Build history of the part. All positions in model axes, mm. A direction names the side the tool comes from. Round coordinates to 2 decimals unless told otherwise and drop trailing zeros. Write each loop counter-clockwise with the first axis right and the second up, starting at its lowest first coordinate (ties: lowest second). Pieces come first, ordered by that corner, then holes. Notation, with made-up numbers: M 53.5,65 L 84.5,65 A12 ccw 84.5,82 Z; hole C -31,39 d8. An arc over 180 degrees is marked long. Write item = value, one per line.
Autodesk Fusion 360 part; units mm, degrees
sketch "Sketch1" plane through (0, 0, 0) normal (0, 1, 0) x (1, 0, 0)
  circle A0 centre (0, 0) radius 12.5
  dimension "d1" = 25
extrude "Extrude1" add sketch "Sketch1" along normal blind 3 makes body 1
chamfer "Chamfer1" distance 3 angle 45 1 edges at (-11.6541, 3, 4.5202) on bodies 1
sketch "Sketch2" plane through (0, 3, 0) normal (0, 1, 0) x (-1, 0, 0)
  circle A0 centre (0, 0) radius 9.5
  circle A1 centre (0, 0) radius 12.5
  dimension "d5" = 25
extrude "Extrude2" add sketch "Sketch2" along normal blind 1 contours A0 | A1 bodies 1
sketch "Sketch3" plane through (0, 0, 0) normal (0, 0, 1) x (1, 0, 0)
  line L0 (0, 0) -> (0.5, 0)
  line L1 (0.5, 0) -> (0.5, 3)
  line L2 (0.5, 3) -> (0, 3)
  line L3 (0, 3) -> (0, 0)
  line L4 (12.5, 3) -> (-12.5, 3)
extrude "Extrude3" add sketch "Sketch3" along normal blind 12.5 separate body makes body 2
chamfer "Chamfer2" distance 2.3 angle 45 1 edges at (0.25, 3, 12.5) on bodies 2
pattern_circular "C-Pattern1" count 6 over 360 about axis through (0, 0, 0) along (0, 1, 0) of bodies 2 makes body 3 at (6.5529, 1, 3.7833) makes body 4 at (6.3029, 1, -4.2163) makes body 5 at (0, 1, -7.5667) makes body 6 at (-6.5529, 1, -3.7833) makes body 7 at (-6.5529, 1, 3.7833)
sketch "Sketch4" plane through (0, 0, 0) normal (0, 0, 1) x (1, 0, 0)
sketch "Sketch5" plane through (0, 0, 0) normal (1, 0, 0) x (0, 0, -1)
  line L0 (0, 0) -> (0.5, 0)
  line L1 (0.5, 0) -> (0.5, 3)
  line L2 (0.5, 3) -> (0, 3)
  line L3 (0, 3) -> (0, 0)
  line L4 (-0.433, 3) -> (4.667, 3)
extrude "Extrude4" add sketch "Sketch5" along normal blind 12.5 separate body makes body 8
chamfer "Chamfer3" distance 1.5 angle 45 1 edges at (12.5, 3, -0.25) on bodies 8
pattern_circular "C-Pattern2" count 3 over 360 about axis through (0, 0, 0) along (0, 1, 0) of bodies 8 makes body 9 at (-4.3497, 1, -6.5339) makes body 10 at (-3.9167, 1, 6.7839)
combine "Combine1" operation add target body 1 tool bodies 7 10 2 6 9 5 4 8 3
sketch "Sketch6" plane through (0, 0, 0) normal (0, -1, 0) x (1, 0, 0)
  arc A0 (10.8253, 6.25) -> (0.5, 12.49) centre (0, 0) ccw
  line L0 (0.5, 12.49) -> (0.5, 12.5)
  line L1 (0.5, 12.5) -> (0, 12.5)
  arc A1 (0, 12.5) -> (-5.812, 11.0667) centre (0, 0) ccw
  line L2 (-5.812, 11.0667) -> (-5.817, 11.0753)
  line L3 (-5.817, 11.0753) -> (-6.25, 10.8253)
  arc A2 (-6.25, 10.8253) -> (-10.5667, 6.678) centre (0, 0) ccw
  line L4 (-10.5667, 6.678) -> (-10.5753, 6.683)
  line L5 (-10.5753, 6.683) -> (-10.8253, 6.25)
  arc A3 (-10.8253, 6.25) -> (-11.0667, -5.812) centre (0, 0) ccw
  line L6 (-11.0667, -5.812) -> (-11.0753, -5.817)
  line L7 (-11.0753, -5.817) -> (-10.8253, -6.25)
  arc A4 (-10.8253, -6.25) -> (-6.678, -10.5667) centre (0, 0) ccw
  line L8 (-6.678, -10.5667) -> (-6.683, -10.5753)
  line L9 (-6.683, -10.5753) -> (-6.25, -10.8253)
  arc A5 (-6.25, -10.8253) -> (-0.5, -12.49) centre (0, 0) ccw
  line L10 (-0.5, -12.49) -> (-0.5, -12.5)
  line L11 (-0.5, -12.5) -> (0, -12.5)
  arc A6 (0, -12.5) -> (10.5667, -6.678) centre (0, 0) ccw
  line L12 (10.5667, -6.678) -> (10.5753, -6.683)
  line L13 (10.5753, -6.683) -> (10.8253, -6.25)
  arc A7 (10.8253, -6.25) -> (12.49, -0.5) centre (0, 0) ccw
  line L14 (12.49, -0.5) -> (12.5, -0.5)
  line L15 (12.5, -0.5) -> (12.5, 0)
  arc A8 (12.5, 0) -> (11.0667, 5.812) centre (0, 0) ccw
  line L16 (11.0667, 5.812) -> (11.0753, 5.817)
  line L17 (11.0753, 5.817) -> (10.8253, 6.25)
scale "Scale1" factor 1.8 about (7.9658, 3, -5.1764) bodies 1
sketch "Sketch7" plane through (0, -2.4, 0) normal (0, -1, 0) x (1, 0, 0)
  arc A0 (13.1129, 15.3911) -> (-5.4727, 26.6231) centre (-6.3727, 4.1411) ccw
  line L0 (-5.4727, 26.6231) -> (-5.4727, 26.6411)
  line L1 (-5.4727, 26.6411) -> (-6.3727, 26.6411)
  arc A1 (-6.3727, 26.6411) -> (-16.8342, 24.0611) centre (-6.3727, 4.1411) ccw
  line L2 (-16.8342, 24.0611) -> (-16.8432, 24.0767)
  line L3 (-16.8432, 24.0767) -> (-17.6227, 23.6267)
  arc A2 (-17.6227, 23.6267) -> (-25.3926, 16.1616) centre (-6.3727, 4.1411) ccw
  line L4 (-25.3926, 16.1616) -> (-25.4082, 16.1706)
  line L5 (-25.4082, 16.1706) -> (-25.8582, 15.3911)
  arc A3 (-25.8582, 15.3911) -> (-26.2926, -6.3204) centre (-6.3727, 4.1411) ccw
  line L6 (-26.2926, -6.3204) -> (-26.3082, -6.3294)
  line L7 (-26.3082, -6.3294) -> (-25.8582, -7.1089)
  arc A4 (-25.8582, -7.1089) -> (-18.3931, -14.8788) centre (-6.3727, 4.1411) ccw
  line L8 (-18.3931, -14.8788) -> (-18.4021, -14.8944)
  line L9 (-18.4021, -14.8944) -> (-17.6227, -15.3444)
  arc A5 (-17.6227, -15.3444) -> (-7.2727, -18.3408) centre (-6.3727, 4.1411) ccw
  line L10 (-7.2727, -18.3408) -> (-7.2727, -18.3589)
  line L11 (-7.2727, -18.3589) -> (-6.3727, -18.3589)
  arc A6 (-6.3727, -18.3589) -> (12.6473, -7.8793) centre (-6.3727, 4.1411) ccw
  line L12 (12.6473, -7.8793) -> (12.6629, -7.8883)
  line L13 (12.6629, -7.8883) -> (13.1129, -7.1089)
  arc A7 (13.1129, -7.1089) -> (16.1093, 3.2411) centre (-6.3727, 4.1411) ccw
  line L14 (16.1093, 3.2411) -> (16.1273, 3.2411)
  line L15 (16.1273, 3.2411) -> (16.1273, 4.1411)
  arc A8 (16.1273, 4.1411) -> (13.5473, 14.6027) centre (-6.3727, 4.1411) ccw
  line L16 (13.5473, 14.6027) -> (13.5629, 14.6117)
  line L17 (13.5629, 14.6117) -> (13.1129, 15.3911)
  circle A9 centre (-6.3727, 4.1411) radius 7.5
  dimension "d19" = 15
extrude "Extrude5" add sketch "Sketch7" along normal blind 10 contours A9 bodies 1
sketch "Sketch8" plane through (0, -12.4, 0) normal (0, -1, 0) x (1, 0, 0)
  circle A0 centre (-6.3727, 4.1411) radius 7.5
  circle A1 centre (-6.3727, 4.1411) radius 2.5
  dimension "d22" = 5
extrude "Extrude6" cut sketch "Sketch8" against normal blind 100 contours A1 bodies 1
sketch "Sketch9" plane through (0, 0, 0) normal (0, 0, 1) x (1, 0, 0)
  circle A0 centre (-6.3727, -6.4827) radius 1.375
  dimension "d25" = 2.75
extrude "Extrude7" add sketch "Sketch9" against normal blind 10 separate body makes body 11
move_body "Move1" bodies 11 to x (1, 0, 0) y (0, 1, 0) z (0, 0, 1) at (0, 0, 4)
combine "Combine2" operation cut target body 1 tool bodies 11
extrude "Extrude8" add 1 faces at (-5.1104, -2.4, -13.2744) along direction (0, -1, 0) blind 0.5 on bodies 1 bodies 1
move_face "OffsetFaces1" offset 3.5 1 faces at (-8.6648, -7.2979, -3) on bodies 1
move_face "OffsetFaces2" offset -0.13 1 faces at (-3.8851, -6.6667, 3.8922) on bodies 1
move_face "OffsetFaces3" offset -0.05 1 faces at (-5.2578, -5.6779, -3.9485) on bodies 1
sketch "Sketch10" plane through (0, 0, 0) normal (0, 0, 1) x (1, 0, 0)
  line L0 (-6.3727, -2.9) -> (12.6473, -2.9)
  line L1 (-3.4477, -6.4827) -> (-3.4477, -2.6827)
  line L2 (-9.2977, -6.4827) -> (-9.2977, -10.2827)
  line L3 (-9.2977, -10.2827) -> (-3.4477, -10.2827)
  line L4 (-3.4477, -10.2827) -> (-3.4477, -2.6827)
  line L5 (-3.4477, -2.6827) -> (-9.2977, -2.6827)
  line L6 (-9.2977, -2.6827) -> (-9.2977, -10.2827)
  dimension "d33" = 1.5
  dimension "d34" = 1.5
  dimension "d36" = 3.8
extrude "Extrude9" add sketch "Sketch10" against normal blind 3.4 separate body makes body 12
extrude "Extrude10" add 1 faces at (-7.3477, -10.2827, -1.1333) along direction (0, -1, 0) blind 5 on bodies 12 bodies 12
combine "Combine3" operation cut target body 1 tool bodies 12 keep tools
hidden bodies 12
1. Band-saw the part on A-A (y = -9.75). List the corners of the cut face in (x, z), plus the area to 3 significant figures.
Responses:
outline = C -6.37,4.14 d22; hole M -9.3,-3.4 L -3.45,-3.4 L -3.45,0 L -9.3,0 Z; hole C -6.37,4.14 d5.26
area = 339 mm²
2. Tool access for faces 1 (the face through (-5.473, 1, 24)), 2 (the face through (-23.87, 0.9, 14.75)), 3 (the face through (-6, -9, 0)), 4 (the face through (-6.682, -7.874, -5.105)), 5 (the face through (14, 1, 3.241)): list every direction of +Z, -Z, +X, -X, +Y, -Y with a clear straight run to the whole face (end or side of a thin tool).
Responses:
face_1 = +Z, +X
face_2 = +Z, -X
face_3 = -Y
face_4 = -Z
face_5 = -Z, +X
3. Probe probe 1 along Y at (x, z) = (8, 13); probe 2 along Y at (x, z) = (8, -7.5); probe 3 along Z at (x, y) = (-8, -11.5) (3 decimals). List the from-to ranges inside material, lowest first.
Responses:
probe_1 = -2.9 to 4.8
probe_2 = -2.9 to 1.61, 3 to 4.8
probe_3 = -6.738 to -3.4, 0 to 2.075, 6.207 to 15.02
4. Flat gauge pins, fed straight in: pin 1 (6.5 mm diameter, centred on x = -5, y = -8, fed in from -Z); pin 2 (2.5 mm diameter, centred on y = 1, z = 25.5, fed in from -X); pin 3 (8 mm diameter, centred on y = -8.5, z = -8.5, fed in from -X); pin 4 (8 mm diameter, centred on x = -9.5, y = -1.5, fed in from +Z). Where does each tip first touch, or does it go through?
Responses:
pin_1 = -6.86
pin_2 = -6.37
pin_3 = -13.18
pin_4 = 26.64
5. Mould opens along X. For faces 6 (the face through (10.937, 0.513, -5.853)), 7 (the face through (-9.298, -7, -2)), 8 (the face through (-12, -2.9, -6)) say: pulls with the +X half, pulls with the -X half, needs draft (parallel to the pull), parting line crosses it, or undercut.
Responses:
face_6 = pulls with the +X half
face_7 = undercut
face_8 = needs draft
